Answer from the drawing. Dimensions are ordinates in mm from the lowest x, y and z of the part. Give positions to 0.01 mm unless a question says otherwise; leave off trailing zeros. Loops run counter-clockwise (first coordinate to the right, second up) from the corner with the lowest first, then second, coordinate; pieces in that order, holes last. Notation, with made-up numbers: (85.25, 47.25) - (122.25, 47.25) arc R28 ccw to (122.25, 65.25) - close; hole circle Ø11 at (33.5, 81). An arc over 180 degrees is marked (long way). Write each question's results on one line, items separated by ' | '. Start each with the question number.
Q1. Given pin 1 (4 mm diameter, centred on x = 71.5, z = 14.5, fed in from +Y); pin 2 (3 mm diameter, centred on x = 49, z = 12.5, fed in from -Y), each flat-ended and moving along its own axis, determine where each tip first touches the part or whether it passes through.
Q2. The part is cut by section A-A, the plane z = 12.5. Write down the section's boundary in (x, y), plus the area to 3 significant figures.
Q3. The part is cut by section B-B, the plane x = 49. Write down the section's boundary in (y, z), plus the area to 3 significant figures.
Q4. Find the intervals of material crossed by line 1 (X direction, y = 1.25, z = 7); line 2 (X direction, y = 0.8, z = 12.5); line 3 (Z direction, x = 71, y = 0.35), in increasing order. Write a range as from..to.
Q5. The part is cut by section C-C, the plane z = 7.75. Write down the section's boundary in (x, y), plus the area to 3 significant figures.
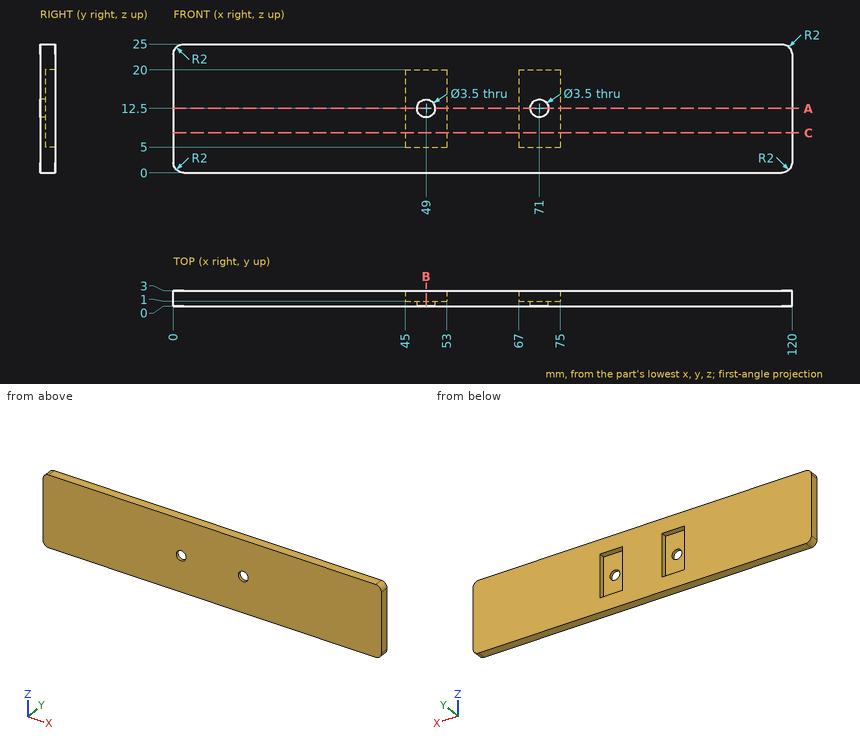
Check sheet entries:
1) pin 1: stops at y = 1 | pin 2: passes through
2) outline: (0, 0) - (47.25, 0) - (47.25, 1) - (45, 1) - (45, 3) - (0, 3) - close; (50.75, 0) - (69.25, 0) - (69.25, 1) - (67, 1) - (67, 3) - (53, 3) - (53, 1) - (50.75, 1) - close; (72.75, 0) - (120, 0) - (120, 3) - (75, 3) - (75, 1) - (72.75, 1) - close | area: 321 mm^2
3) outline: (0, 0) - (3, 0) - (3, 5) - (1, 5) - (1, 10.75) - (0, 10.75) - close; (0, 14.25) - (1, 14.25) - (1, 20) - (3, 20) - (3, 25) - (0, 25) - close | area: 41.5 mm^2
4) line 1: x = 0..45, 53..67, 75..120 | line 2: x = 0..47.25, 50.75..69.25, 72.75..120 | line 3: z = 0..10.75, 14.25..25
5) outline: (0, 0) - (120, 0) - (120, 3) - (75, 3) - (75, 1) - (67, 1) - (67, 3) - (53, 3) - (53, 1) - (45, 1) - (45, 3) - (0, 3) - close | area: 328 mm^2
